```python
from build123d import *

# Parameters (mm, degrees)
ESQUISSE1_W                                    = 20
ESQUISSE1_H                                    = 20
BOSS_EXTRU_1_DEPTH                             = 3.2
CONG_1_R                                       = 1.8
DIAM_TRE_DU_PER_AGE_1_0_1_1_D                  = 1
ESQUISSE4_W                                    = 10.2
ESQUISSE4_H                                    = 7.8
ENL_V_MAT_EXTRU_1_DEPTH                        = 0.7
ESQUISSE5_W                                    = 10.2
ESQUISSE5_H                                    = 5.1
ENL_V_MAT_EXTRU_2_DEPTH                        = 1
CONG_2_R                                       = 1
FRAISAGE_POUR_VIS_T_TE_FRAIS_E_M21_D           = 2.2
FRAISAGE_POUR_VIS_T_TE_FRAIS_E_M21_CSINK_D     = 4.4
FRAISAGE_POUR_VIS_T_TE_FRAIS_E_M21_CSINK_ANGLE = 90
ESQUISSE8_R                                    = 4
ENL_V_MAT_EXTRU_3_DEPTH                        = 15.499655168


with BuildPart() as part:
    # Esquisse1 → Boss.-Extru.1 (new body)
    with BuildSketch(Plane.XY):
        Rectangle(ESQUISSE1_W, ESQUISSE1_H)
    extrude(amount=BOSS_EXTRU_1_DEPTH)

    # Congé1
    cong_1_edges = [part.edges().sort_by_distance(p)[0] for p in [
        (-10, 10, 1.6),
        (10, 10, 1.6),
        (10, -10, 1.6),
        (-10, -10, 1.6),
    ]]
    fillet(cong_1_edges, radius=CONG_1_R)

    # Diamètre du perçage Ø1.0 (1)1 (through all)
    with Locations(Plane.XY.offset(3.2)):
        with Locations((3.1, -5), (3.4, 0), (5.5, 1.85), (-5.5, 1.85), (-3.4, 0), (-3.1, -5)):
            Hole(DIAM_TRE_DU_PER_AGE_1_0_1_1_D / 2)

    # Esquisse4 → Enlèv. mat.-Extru.1 (cut)
    with BuildSketch(Plane.XY.offset(3.2)):
        with Locations((0, -6.1)):
            Rectangle(ESQUISSE4_W, ESQUISSE4_H)
    extrude(amount=-ENL_V_MAT_EXTRU_1_DEPTH, mode=Mode.SUBTRACT)

    # Esquisse5 → Enlèv. mat.-Extru.2 (cut)
    with BuildSketch(Plane.XY.offset(2.5)):
        with Locations((0, -4.75)):
            Rectangle(ESQUISSE5_W, ESQUISSE5_H)
    extrude(amount=-ENL_V_MAT_EXTRU_2_DEPTH, mode=Mode.SUBTRACT)

    # Congé2
    cong_2_edges = [part.edges().sort_by_distance(p)[0] for p in [
        (-5.1, -2.2, 2.35),
        (5.1, -2.2, 2.35),
        (-5.1, -7.3, 2),
        (5.1, -7.3, 2),
    ]]
    fillet(cong_2_edges, radius=CONG_2_R)

    # Fraisage pour vis à tête fraisée M21 (through all)
    with Locations(Plane.XY.offset(3.2)):
        with Locations((-7.5, 7.5), (-7.5, -7.5), (7.5, -7.5), (7.5, 7.5)):
            CounterSinkHole(FRAISAGE_POUR_VIS_T_TE_FRAIS_E_M21_D / 2, FRAISAGE_POUR_VIS_T_TE_FRAIS_E_M21_CSINK_D / 2, counter_sink_angle=FRAISAGE_POUR_VIS_T_TE_FRAIS_E_M21_CSINK_ANGLE)

    # Esquisse8 → Enlèv. mat.-Extru.3 (cut, through all)
    with BuildSketch(Plane.XY.offset(3.2)):
        with Locations((0, 12.2)):
            Circle(ESQUISSE8_R)
    extrude(amount=-ENL_V_MAT_EXTRU_3_DEPTH, mode=Mode.SUBTRACT)


solid = part.part
```
Input: part model. Units: mm. Frame: model coordinates. A direction names the side the tool comes from. Coordinates: 2 decimals unless noted, no trailing zeros. Loops run counter-clockwise (first coordinate to the right, second up) from the corner with the lowest first, then second, coordinate; pieces in that order, holes last.
Q1. Mould query, pull axis X, two halves, no side actions, for faces 3 (the flat face through (0, 0, 0)), 4 (the cylindrical face through (9.459, -9.487, 1.622)), 5 (the flat face through (0, -7.3, 2)). Classes: +X half, -X half, draft (parallel to the pull), parting line (faces both ways), or undercut.
Results are:
face 3: draft
face 4: +X half
face 5: undercut
Q2. Line query: line 1 along Y through (x, z) = (-3.4, 2.35); line 2 along X through (y, z) = (-7.5, 1.6); line 3 along Y through (x, z) = (-5.5, 2). Output: solid intervals per line, ascending.
Results are:
line 1: y = -10 to -7.3, -2.2 to -0.5, 0.5 to 10
line 2: x = -10 to -8.6, -6.4 to 6.4, 8.6 to 10
line 3: y = -10 to 1.35, 2.35 to 10
Q3. Contact query for flat-ended pins moving along their axis: pin 1 (2.5 mm diameter, centred on x = 7.5, y = -7.5, fed in from +Z); pin 2 (1.8 mm diameter, centred on x = -2, y = -7.5, fed in from +Z); pin 3 (0.8 mm diameter, centred on x = 1, z = 2, fed in from +Y); pin 4 (1.3 mm diameter, centred on x = -7.5, y = 7.5, fed in from -Z). Output: stop coordinate, or through.
Results are:
pin 1: stops at z = 2.25
pin 2: stops at z = 2.5
pin 3: stops at y = 8.45
pin 4: passes through
Q4. Section D-D, the plane y = 1.85. Return the cut outline in (x, z).
Results are:
outline: (-10, 0) - (-6, 0) - (-6, 3.2) - (-10, 3.2) - close; (-5, 0) - (5, 0) - (5, 3.2) - (-5, 3.2) - close; (6, 0) - (10, 0) - (10, 3.2) - (6, 3.2) - close
Q5. Section C-C, the plane z = 1.2. Give the number of separate pieces and of enclosed holes in the cut face, and give its area (3 significant figures).
Results are:
separate pieces: 1
enclosed holes: 10
area: 369 mm2
Q6. Section A-A, the plane x = 7.5. Return the cut outline in (y, z), and give its area (3 significant figures).
Results are:
outline: (-10, 0) - (-8.6, 0) - (-8.6, 2.1) - (-9.7, 3.2) - (-10, 3.2) - close; (-6.4, 0) - (6.4, 0) - (6.4, 2.1) - (5.3, 3.2) - (-5.3, 3.2) - (-6.4, 2.1) - close; (8.6, 0) - (10, 0) - (10, 3.2) - (9.7, 3.2) - (8.6, 2.1) - close
area: 47.5 mm2
Q7. Set-up query: faces 1 (the flat face through (5.1, -6, 3)), 2 (the flat face through (-6, 10, 2)). Return all of +Z, -Z, +X, -X, +Y, -Y with unobstructed straight access to the full face (end or side cutting, diameter ignored); none if empty.
Results are:
face 1: +Z
face 2: +Z, -Z, +X, -X, +Y
